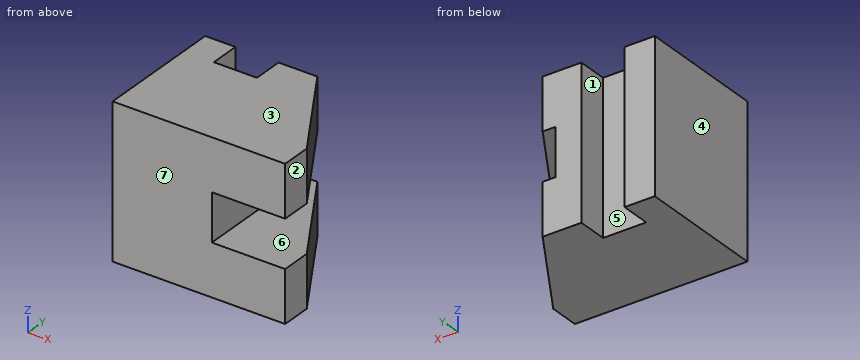
from build123d import *

# Parameters (mm, degrees)
Y_KSEKLIK_EKSTR_ZYON1_DEPTH = 70
IZIM2_OUTSIDE_W             = 106.414
IZIM2_OUTSIDE_H             = 96.414
KES_EKSTR_ZYON3_DEPTH       = 60


with BuildPart() as part:
    # Çizim1 → Yükseklik-Ekstrüzyon1 (new body)
    with BuildSketch(Plane.XY):
        Polygon((0, 0), (0, 60), (14, 60), (14, 46), (34, 46), (34, 60), (52, 60), (80, 14), (80, 0), align=None)
    extrude(amount=-Y_KSEKLIK_EKSTR_ZYON1_DEPTH)

    # Çizim2 outside → Kes-Ekstrüzyon3 (cut)
    with BuildSketch(Plane(origin=(0, 0, 0), x_dir=(1, 0, 0), z_dir=(0, 1, 0))):
        with Locations((40, 35)):
            Rectangle(IZIM2_OUTSIDE_W, IZIM2_OUTSIDE_H)
        Polygon((80, 70), (46, 70), (0, 70), (0, 0), (80, 0), (80, 24), (46, 24), (46, 46), (80, 46), align=None, mode=Mode.SUBTRACT)
    extrude(amount=KES_EKSTR_ZYON3_DEPTH, mode=Mode.SUBTRACT)


solid = part.part
Can you work these out from the model? Positions are in its coordinate system, mm. Face numbers are marked on the shaded views. A direction names the side the tool comes from. Give positions to 0.01 mm unless a question says otherwise; leave off trailing zeros. Loops run counter-clockwise (first coordinate to the right, second up) from the corner with the lowest first, then second, coordinate; pieces in that order, holes last. Notation, with made-up numbers: (0, 4.25) - (44, 4.25) arc R12 ccw to (44, 17.25) - close; hole circle Ø5 at (56.5, 23). An arc over 180 degrees is marked (long way). Return JSON: item names as keys, results as strings.
1. I want a section at A-A on x = 48. Please give me the cut outline in (y, z), and give its area (3 significant figures).
Output values:
{"outline": "(0, -70) - (60, -70) - (60, -46) - (0, -46) - close; (0, -24) - (60, -24) - (60, 0) - (0, 0) - close", "area": "2,880 mm²"}
2. I want a section at D-D on y = 25.5. Please give me the cut outline in (x, z).
Output values:
{"outline": "(0, -70) - (73, -70) - (73, -46) - (46, -46) - (46, -24) - (73, -24) - (73, 0) - (0, 0) - close"}
3. If I drill on line 1 (X direction, y = 13.5, z = -33); line 2 (Z direction, x = 54, y = 3), over which ranges is the centre line in solid material (lowest first)?
Output values:
{"line 1": "x = 0 to 46", "line 2": "z = -70 to -46, -24 to 0"}
4. We'd pull the mould along X, two halves only. Please class the marked faces 1, 2, 3 and 4: +X half, -X half, draft (parallel to the pull), parting line (faces both ways), or undercut.
Output values:
{"face 1": "undercut", "face 2": "+X half", "face 3": "draft", "face 4": "-X half"}
5. For the marked faces 5, 6 and 7, which set-ups out of +Z, -Z, +X, -X, +Y, -Y let a thin tool reach every point of the face, with its end or its side?
Output values:
{"face 5": "+Z, -Z, +Y", "face 6": "+X, +Y, -Y", "face 7": "+Z, -Z, +X, -X, -Y"}
6. I'm going to push flat-ended pins straight in: pin 1 Ø4 at (x, z) = (23, -44.5) entering from +Y; pin 2 Ø4 at (y, z) = (54, -41.5) entering from +X; pin 3 Ø24 at (y, z) = (42, -37) entering from +X. Where does each tip first touch, or does it pass through?
Output values:
{"pin 1": "stops at y = 46", "pin 2": "stops at x = 46", "pin 3": "stops at x = 67.79"}
7. I want a section at C-C on y = 49.5. Please give me the cut outline in (x, z).
Output values:
{"outline": "(0, -70) - (14, -70) - (14, 0) - (0, 0) - close; (34, -70) - (58.39, -70) - (58.39, -46) - (46, -46) - (46, -24) - (58.39, -24) - (58.39, 0) - (34, 0) - close"}
8. I want a section at B-B on z = -53.5. Please give me the cut outline in (x, y), and give its area (3 significant figures).
Output values:
{"outline": "(0, 0) - (80, 0) - (80, 14) - (52, 60) - (34, 60) - (34, 46) - (14, 46) - (14, 60) - (0, 60) - close", "area": "3,880 mm²"}
